```python
from build123d import *

# Parameters (mm, degrees)
F0_W          = 127
F0_H          = 25.4
F1_DEPTH      = 0.762
F2_DEPTH      = 12.7
F3_W          = 22.5780475885
F3_H          = 24.1802637465
F4_DEPTH      = 101.6
F4_DEPTH_BACK = 101.6
F5_R          = 3.429
F6_DEPTH      = 25.4


with BuildPart() as f1:
    # F0 (on Top) → F1 (new body)
    with BuildSketch(Plane.XY):
        Rectangle(F0_W, F0_H)
    extrude(amount=F1_DEPTH)

    # F0 (on Top) → F2 (join)
    with BuildSketch(Plane.XY):
        Rectangle(F0_W, F0_H)
    extrude(amount=F2_DEPTH)

    # F3 (on Right) → F4 (cut, two sides)
    with BuildSketch(Plane.YZ) as f4_sk:
        with Locations((0, 12.7019658685)):
            Rectangle(F3_W, F3_H)
    extrude(amount=-F4_DEPTH, mode=Mode.SUBTRACT)
    extrude(f4_sk.sketch, amount=F4_DEPTH_BACK, mode=Mode.SUBTRACT)

    # F5 (on face) → F6 (cut)
    with BuildSketch(Plane.XY.offset(0.6118339952)):
        Circle(F5_R)
        with Locations((-53.594, 0)):
            Circle(F5_R)
        with BuildLine():
            Line((-22.479, 3.429), (-35.814, 3.429))
            ThreePointArc((-35.814, 3.429), (-39.243, 0), (-35.814, -3.429))
            Line((-35.814, -3.429), (-22.479, -3.429))
            ThreePointArc((-22.479, -3.429), (-19.05, 0), (-22.479, 3.429))
        make_face()
        with BuildLine():
            ThreePointArc((35.814, -3.429), (39.243, 0), (35.814, 3.429))
            Line((35.814, 3.429), (22.479, 3.429))
            ThreePointArc((22.479, 3.429), (19.05, 0), (22.479, -3.429))
            Line((22.479, -3.429), (35.814, -3.429))
        make_face()
        with Locations((53.594, 0)):
            Circle(F5_R)
    extrude(amount=-F6_DEPTH, mode=Mode.SUBTRACT)


solid = f1.part
```
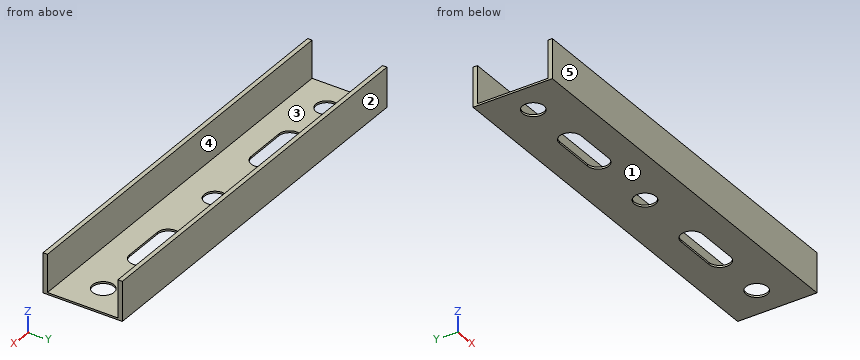
Check sheet for the modelled part. Datum: model origin and axes. Units: mm. Face numbers are marked on the shaded views. A direction names the side the tool comes from. Round coordinates to 2 decimals unless told otherwise and drop trailing zeros. Loops run counter-clockwise (first coordinate to the right, second up) from the corner with the lowest first, then second, coordinate; pieces in that order, holes last. Notation, with made-up numbers: M 42.25,35.5 L 100.25,35.5 A19 ccw 100.25,58.5 Z; hole C 17.5,12 d9. An arc over 180 degrees is marked long. Answer as a JSON object with one key per item and string values.
1. Scan lines: line 1 (Y direction, x = 12, z = 4.5); line 2 (Y direction, x = -27, z = 0.5); line 3 (Z direction, x = 12, y = -11). Record each from-to range of solid material in increasing order.
Reply:
{"line 1": "y = -12.7 to -11.29, 11.29 to 12.7", "line 2": "y = -12.7 to -3.43, 3.43 to 12.7", "line 3": "z = 0 to 0.61"}
2. Section check D-D (x = -46.5). Record the boundary of the cut face in (y, z).
Reply:
{"outline": "M -12.7,0 L 12.7,0 L 12.7,12.7 L 11.29,12.7 L 11.29,0.61 L -11.29,0.61 L -11.29,12.7 L -12.7,12.7 Z"}
3. Section check C-C (z = 5). Record the boundary of the cut face in (x, y).
Reply:
{"outline": "M -63.5,-12.7 L 63.5,-12.7 L 63.5,-11.29 L -63.5,-11.29 Z; M -63.5,11.29 L 63.5,11.29 L 63.5,12.7 L -63.5,12.7 Z"}
4. Gauge pin test, flat end, axial feed: P1, Ø11, axis at x = 53.594, y = 0, coming from the +Z side. Record the tip position at first contact, or that the pin passes through.
Reply:
{"P1": "stops at z = 0.61"}
5. Mould release check, pull along Y, two halves, no side actions. Record for the marked faces 1, 2 and 3: pulls with the +Y half, pulls with the -Y half, needs draft (parallel to the pull), parting line crosses it, or undercut.
Reply:
{"face 1": "needs draft", "face 2": "pulls with the +Y half", "face 3": "undercut"}
6. Section check B-B (y = 0). Record the boundary of the cut face in (x, z) (3 decimals).
Reply:
{"outline": "M -63.5,0 L -57.023,0 L -57.023,0.612 L -63.5,0.612 Z; M -50.165,0 L -39.243,0 L -39.243,0.612 L -50.165,0.612 Z; M -19.05,0 L -3.429,0 L -3.429,0.612 L -19.05,0.612 Z; M 3.429,0 L 19.05,0 L 19.05,0.612 L 3.429,0.612 Z; M 39.243,0 L 50.165,0 L 50.165,0.612 L 39.243,0.612 Z; M 57.023,0 L 63.5,0 L 63.5,0.612 L 57.023,0.612 Z"}
7. Access from +Z, -Z, +X, -X, +Y, -Y to the whole of each face (thin tool, end or side, straight path). Record for the marked faces 4 and 5.
Reply:
{"face 4": "+Z, +X, -X", "face 5": "+Z, -Z, +X, -X, -Y"}
8. Section check A-A (x = 0). Record the boundary of the cut face in (y, z).
Reply:
{"outline": "M -12.7,0 L -3.43,0 L -3.43,0.61 L -11.29,0.61 L -11.29,12.7 L -12.7,12.7 Z; M 3.43,0 L 12.7,0 L 12.7,12.7 L 11.29,12.7 L 11.29,0.61 L 3.43,0.61 Z"}
